Source: three-view drawing plus pictorial views. Frame: mm from the lowest corner of the part. Give positions to 0.01 mm unless a question says otherwise; leave off trailing zeros. Order: outer loops, then holes, each group sorted by start corner. A loop starts at its lowest first (then second) coordinate and runs counter-clockwise, first axis right, second up. Notation, with made-up numbers: M -35.75,58 L -12.75,58 A26 cw -12.75,84 Z; hole C 13.5,-13.5 d4. An arc over 180 degrees is marked long. Use CSV: the item, a comma, the result in double quotes.
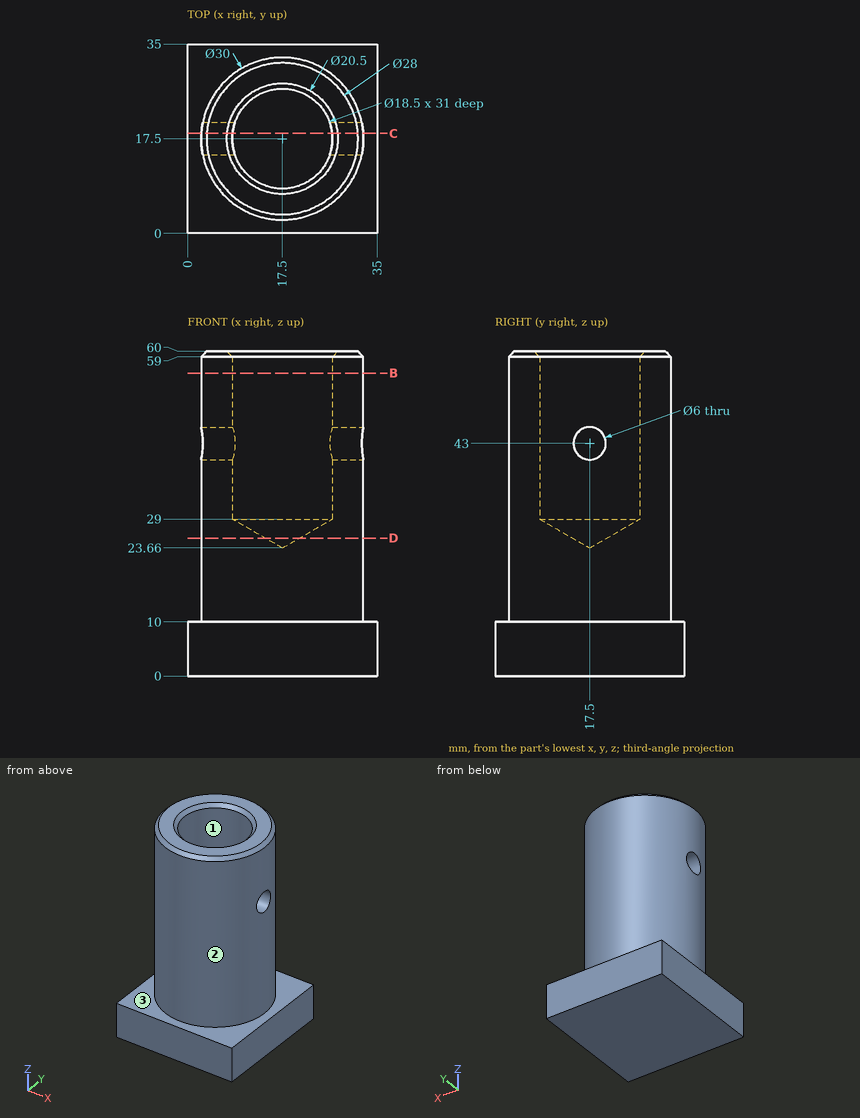
1. Pin query (flat end, axial travel): pin 1 Ø1 at (y, z) = (14, 12.5) entering from -X; pin 2 Ø5 at (y, z) = (17.5, 43) entering from +X; pin 3 Ø7 at (y, z) = (17.5, 43) entering from +X; pin 4 Ø1.5 at (x, z) = (13, 34) entering from +Y. Return the tip coordinate at first contact, or that it passes through.
Answer:
pin 1,"x = 2.8"
pin 2,"through"
pin 3,"x = 32.5"
pin 4,"y = 32.02"
2. Line query: line 1 (Y direction, x = 17, z = 42); line 2 (Y direction, x = 15.5, z = 37.5) (1 decimal); line 3 (Z direction, x = 16.5, y = 2). Output: solid intervals per line, ascending.
Answer:
line 1,"2.51 to 8.26, 26.74 to 32.49"
line 2,"2.6 to 8.5, 26.5 to 32.4"
line 3,"0 to 10"
3. Pull-direction query (Y, two-part tool) for the marked faces 1, 2 and 3; classes: +Y half, -Y half, draft (parallel to the pull), parting line (faces both ways), or undercut.
Answer:
face 1,"undercut"
face 2,"parting line"
face 3,"draft"
4. Section D-D, the plane z = 25.5. Return the cut outline in (x, y) (1 decimal).
Answer:
outline,"C 17.5,17.5 d30; hole C 17.5,17.5 d6.4"
5. Section C-C, the plane y = 18.5. Give the number of separate pieces and of enclosed holes in the cut face, plus the area to 3 significant figures.
Answer:
separate pieces,"3"
enclosed holes,"0"
area,"1,160 mm2"
6. Section B-B, the plane z = 56. Return the cut outline in (x, y).
Answer:
outline,"C 17.5,17.5 d30; hole C 17.5,17.5 d18.5"
